Can you work these out from the drawing? Everything is in mm from the part's minimum corner. A direction names the side the tool comes from. Coordinates: 2 decimals unless noted, no trailing zeros. Write each loop counter-clockwise with the first axis right and the second up, starting at its lowest first coordinate (ties: lowest second). Pieces come first, ordered by that corner, then holes. Notation, with made-up numbers: (25, 43) -> (42, 43) arc R15 ccw to (42, 53) -> close; hole circle Ø4 at (-17, 30). An arc over 180 degrees is marked (long way). Use a Markdown table: item, result. Add a question column.
Item 1: On a 3-axis mill with a long thin cutter (end or side, diameter ignored), from which of +Z, -Z, +X, -X, +Y, -Y can I reach the whole of each face in a straight line? I mean the marked faces 4 and 5. Say none if no direction works.
Item 2: Imagine slicing it at B-B, the plane z = 23.5. Write out the boundary of the cut face in (x, y), and give its area (3 significant figures).
Item 3: If we mould it in two halves opening along Z, with no side actions, what happens to the marked faces 1, 2 and 3? For each: pulls with the +Z half, pulls with the -Z half, needs draft (parallel to the pull), parting line crosses it, or undercut.
Item 4: If I drill on line 1 along X through (y, z) = (5.5, 34.5); line 2 along Y through (x, z) = (31, 5); line 3 along Z through (x, y) = (8, 5.5), over which ranges is the centre line in solid material (lowest first)? Write a range as from..to.
Item 5: Imagine slicing it at D-D, the plane x = 7. Write out the boundary of the cut face in (y, z), and give its area (3 significant figures).
Item 6: Imagine slicing it at A-A, the plane x = 22. Write out the boundary of the cut face in (y, z).
Item 7: Will these pins go through, and if not, where does the flat tip stop? pin 1 Ø4 at (x, y) = (6, 4) entering from -Z; pin 2 Ø1.7 at (x, y) = (31, 4) entering from +Z; pin 3 Ø4 at (y, z) = (4.5, 23) entering from +X; pin 4 Ø1.7 at (x, y) = (30.5, 4.5) entering from -Z.
Item 8: Imagine slicing it at C-C, the plane y = 1.5. Write out the boundary of the cut face in (x, z), and give its area (3 significant figures).
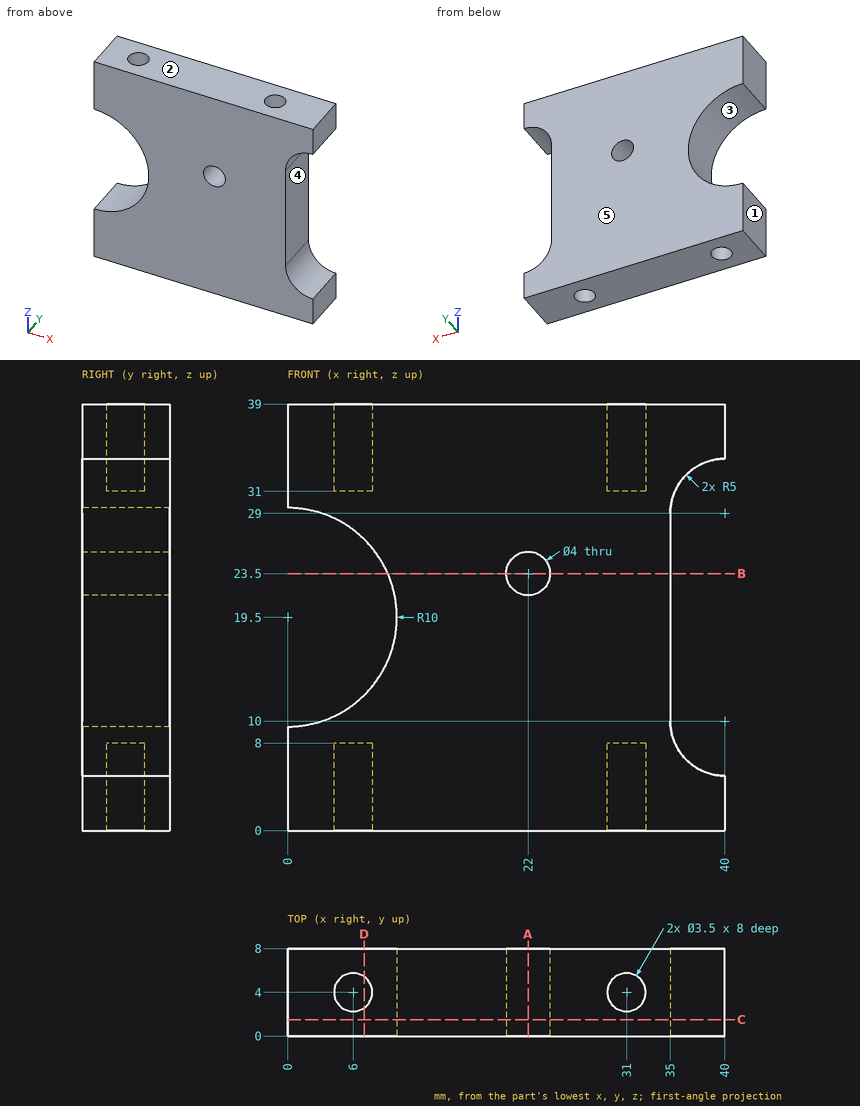
Ans:
| question | item | result |
|---|---|---|
| 1 | face 4 | +X, +Y, -Y |
| 1 | face 5 | +Z, -Z, +X, -X, +Y |
| 2 | outline | (9.17, 0) -> (20, 0) -> (20, 8) -> (9.17, 8) -> close; (24, 0) -> (35, 0) -> (35, 8) -> (24, 8) -> close |
| 2 | area | 175 mm^2 |
| 3 | face 1 | needs draft |
| 3 | face 2 | pulls with the +Z half |
| 3 | face 3 | undercut |
| 4 | line 1 | x = 0..5.1, 6.9..30.1, 31.9..40 |
| 4 | line 2 | y = 0..2.25, 5.75..8 |
| 4 | line 3 | z = 0..13.5, 25.5..39 |
| 5 | outline | (0, 0) -> (2.56, 0) -> (2.56, 8) -> (5.44, 8) -> (5.44, 0) -> (8, 0) -> (8, 12.36) -> (0, 12.36) -> close; (0, 26.64) -> (8, 26.64) -> (8, 39) -> (5.44, 39) -> (5.44, 31) -> (2.56, 31) -> (2.56, 39) -> (0, 39) -> close |
| 5 | area | 152 mm^2 |
| 6 | outline | (0, 0) -> (8, 0) -> (8, 21.5) -> (0, 21.5) -> close; (0, 25.5) -> (8, 25.5) -> (8, 39) -> (0, 39) -> close |
| 7 | pin 1 | stops at z = 0 |
| 7 | pin 2 | stops at z = 31 |
| 7 | pin 3 | stops at x = 35 |
| 7 | pin 4 | stops at z = 8 |
| 8 | outline | (0, 0) -> (40, 0) -> (40, 5) arc R5 cw to (35, 10) -> (35, 29) arc R5 cw to (40, 34) -> (40, 39) -> (0, 39) -> (0, 29.5) arc R10 cw to (0, 9.5) -> close; hole circle Ø4 at (22, 23.5) |
| 8 | area | 1,260 mm^2 |
